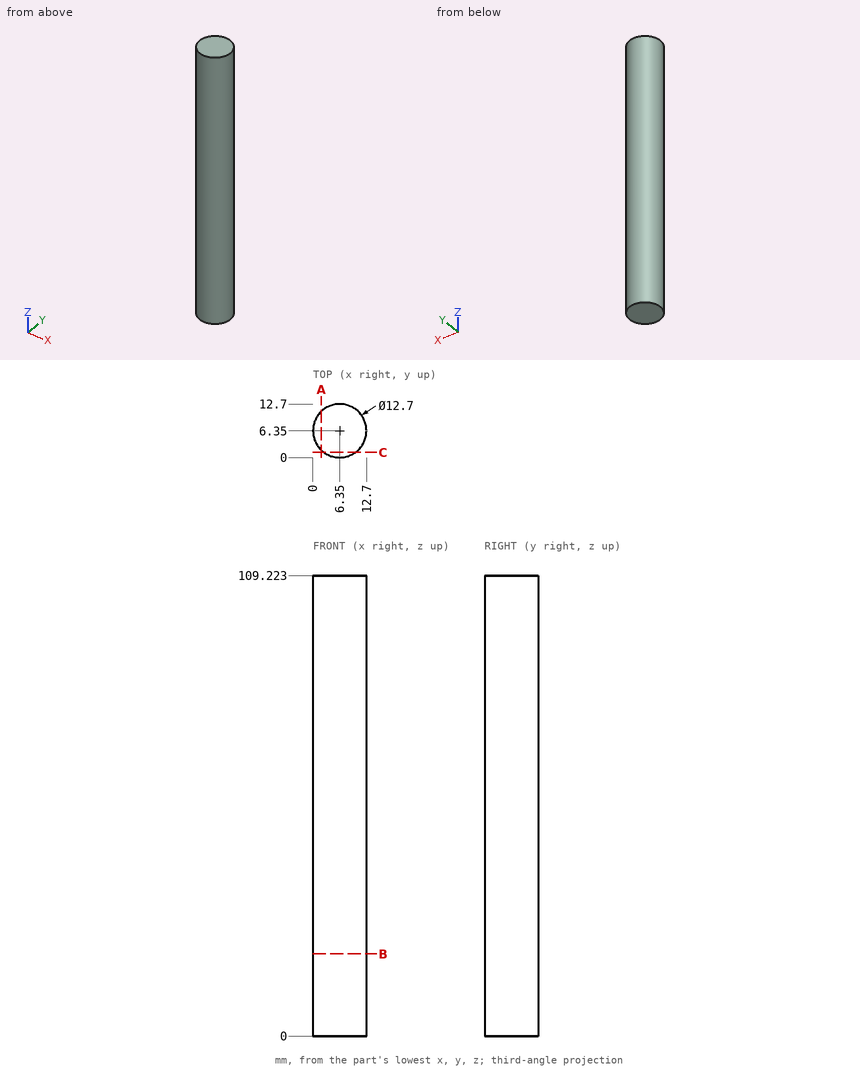
Design review of the part shown in the three views and the two pictorial views. Dimensions are in mm from the part's minimum x, y and z. Round coordinates to 2 decimals unless told otherwise and drop trailing zeros. Write each loop counter-clockwise with the first axis right and the second up, starting at its lowest first coordinate (ties: lowest second). Pieces come first, ordered by that corner, then holes. Notation, with made-up numbers: M 63,41 L 118,41 A35 ccw 118,78 Z; hole C 45.25,76 d7. An arc over 180 degrees is marked long. Use a Markdown table: item, result. Add a question column.
Q1. We need section B-B, the plane z = 19.5. State the section outline as (x, y) points, plus the area to 3 significant figures.
Q2. We need section A-A, the plane x = 2. State the section outline as (y, z) points.
Q3. We need section C-C, the plane y = 1.25. State the section outline as (x, z) points, plus the area to 3 significant figures.
Q4. To check wall thickness, follow line 1 (X direction, y = 6, z = 90); line 2 (X direction, y = 2.75, z = 20); line 3 (Y direction, x = 9.5, z = 76). State the ranges of each line that lie inside material, in increasing order.
Q5. Insertion check: pin 1 (2 mm diameter, centred on y = 8.5, z = 28.5, fed in from -X) (3 decimals); pin 2 (4 mm diameter, centred on x = 8.5, z = 54.5, fed in from -Y); pin 3 (2 mm diameter, centred on x = 4, z = 81.5, fed in from +Y) (3 decimals). Each pin has a flat end and moves straight along its axis. Give the tip position at first contact, or say it passes through.
Findings below:
| question | item | result |
|---|---|---|
| 1 | outline | C 6.35,6.35 d12.7 |
| 1 | area | 127 mm² |
| 2 | outline | M 1.72,0 L 10.98,0 L 10.98,109.22 L 1.72,109.22 Z |
| 3 | outline | M 2.57,0 L 10.13,0 L 10.13,109.22 L 2.57,109.22 Z |
| 3 | area | 826 mm² |
| 4 | line 1 | x = 0.01 to 12.69 |
| 4 | line 2 | x = 1.12 to 11.58 |
| 4 | line 3 | y = 0.84 to 11.86 |
| 5 | pin 1 | stops at x = 0.105 |
| 5 | pin 2 | stops at y = 0 |
| 5 | pin 3 | stops at y = 12.555 |
